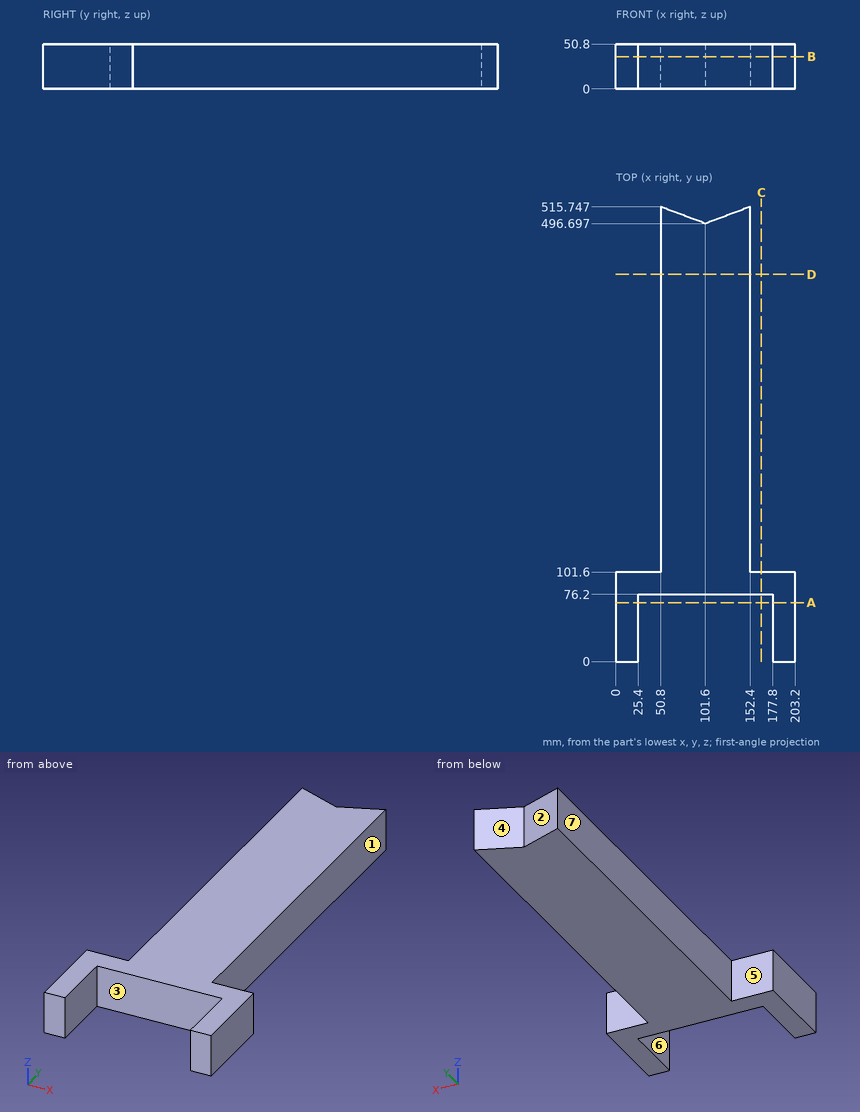
Here's the drawing with two shaded views (mm, measured from the low corner). I have some questions. A direction names the side the tool comes from. Coordinates: 2 decimals unless noted, no trailing zeros. Loops run counter-clockwise (first coordinate to the right, second up) from the corner with the lowest first, then second, coordinate; pieces in that order, holes last. Notation, with made-up numbers: (31.5, 33.25) -> (89.5, 33.25) arc R30 ccw to (89.5, 59.25) -> close; hole circle Ø5 at (-32.5, -33). An arc over 180 degrees is marked (long way). Answer in a Markdown table with one row per item.
(1) Thinking about a two-plate mould opening in X: for the marked faces 4, 5, 6 and 7, which applies, released by +X, released by -X, zero draft, split by the parting line, or undercut?
Results found:
| item | result |
|---|---|
| face 4 | undercut |
| face 5 | zero draft |
| face 6 | undercut |
| face 7 | released by -X |
(2) For the marked faces 1, 2 and 3, which set-ups out of +Z, -Z, +X, -X, +Y, -Y let a thin tool reach every point of the face, with its end or its side?
Results found:
| item | result |
|---|---|
| face 1 | +Z, -Z, +X, +Y |
| face 2 | +Z, -Z, +Y |
| face 3 | +Z, -Z, -Y |
(3) Imagine slicing it at B-B (z = 36.5). List the corners of the cut face in (x, y) for me, plus the area to 3 significant figures.
Results found:
| item | result |
|---|---|
| outline | (0, 0) -> (25.4, 0) -> (25.4, 76.2) -> (177.8, 76.2) -> (177.8, 0) -> (203.2, 0) -> (203.2, 101.6) -> (152.4, 101.6) -> (152.4, 515.75) -> (101.6, 496.7) -> (50.8, 515.75) -> (50.8, 101.6) -> (0, 101.6) -> close |
| area | 50,100 mm^2 |
(4) Imagine slicing it at D-D (y = 439). List the corners of the cut face in (x, z) for me, plus the area to 3 significant figures.
Results found:
| item | result |
|---|---|
| outline | (50.8, 0) -> (152.4, 0) -> (152.4, 50.8) -> (50.8, 50.8) -> close |
| area | 5,160 mm^2 |
(5) Imagine slicing it at C-C (x = 165). List the corners of the cut face in (y, z) for me.
Results found:
| item | result |
|---|---|
| outline | (76.2, 0) -> (101.6, 0) -> (101.6, 50.8) -> (76.2, 50.8) -> close |
(6) Will these pins go through, and if not, where does the flat tip stop? pin 1 Ø15 at (x, z) = (179.5, 20) entering from +Y; pin 2 Ø10 at (y, z) = (138, 20) entering from -X; pin 3 Ø8 at (y, z) = (349, 31.5) entering from +X.
Results found:
| item | result |
|---|---|
| pin 1 | stops at y = 101.6 |
| pin 2 | stops at x = 50.8 |
| pin 3 | stops at x = 152.4 |
(7) Imagine slicing it at A-A (y = 67). List the corners of the cut face in (x, z) for me.
Results found:
| item | result |
|---|---|
| outline | (0, 0) -> (25.4, 0) -> (25.4, 50.8) -> (0, 50.8) -> close; (177.8, 0) -> (203.2, 0) -> (203.2, 50.8) -> (177.8, 50.8) -> close |
(8) If I drill on probe 1 along X at (y, z) = (54, 14); probe 2 along Y at (x, z) = (20, 21.5); probe 3 along X at (y, z) = (125.5, 46), over which ranges is the centre line in solid material (lowest first)?
Results found:
| item | result |
|---|---|
| probe 1 | x = 0 to 25.4, 177.8 to 203.2 |
| probe 2 | y = 0 to 101.6 |
| probe 3 | x = 50.8 to 152.4 |
